Work out the finished part from the listing and answer in its coordinate system (mm). A direction names the side the tool comes from. Coordinates: 2 decimals unless noted, no trailing zeros. Loops run counter-clockwise (first coordinate to the right, second up) from the corner with the lowest first, then second, coordinate; pieces in that order, holes last. Notation, with made-up numbers: (7.25, -34.5) -> (18.25, -34.5) arc R22 ccw to (18.25, -16.5) -> close; hole circle Ø6 at (85.5, 56). An arc over 180 degrees is marked (long way). Use a Markdown table: item, result.
from build123d import *

# Parameters (mm, degrees)
F2_DEPTH = 5
F3_DEPTH = 5
F5_COUNT = 20
F5_ANGLE = 342


with BuildPart() as f2:
    # F1 (on Front) → F2 (new body)
    with BuildSketch(Plane.XZ):
        with BuildLine():
            ThreePointArc((18.791765015, -0.2801004202), (18.7933305583, -0.140054099), (18.7938524157, 0))
            ThreePointArc((18.7938524157, 0), (18.7238802654, 1.6202457939), (18.5144848465, 3.2284267827))
            ThreePointArc((18.5144848465, 3.2284267827), (-18.7354346217, -1.4806681458), (18.791765015, -0.2801004202))
        make_face()
    extrude(amount=F2_DEPTH)

    # F1 (on Front) → F3 (join)
    with BuildSketch(Plane.XZ):
        with BuildLine():
            ThreePointArc((18.5144848465, 3.2284267827), (18.7238802654, 1.6202457939), (18.7938524157, 0))
            ThreePointArc((18.7938524157, 0), (18.7933305583, -0.140054099), (18.791765015, -0.2801004202))
            ThreePointArc((18.791765015, -0.2801004202), (20.4674995965, 0.1731452079), (21.9757526216, 1.0326164403))
            ThreePointArc((21.9757526216, 1.0326164403), (21.9316163904, 1.7332635421), (21.8651473224, 2.4321456718))
            ThreePointArc((21.8651473224, 2.4321456718), (20.2406124153, 3.0440315456), (18.5144848465, 3.2284267827))
        make_face()
    extrude(amount=F3_DEPTH)

    # F5: F2 ×20 about axis
    f5_axis = Axis((0, 6.1465417966, 0), (0, 1, 0))


with BuildPart() as f2_1:
    add(f2.part)
    for i in range(1, F5_COUNT):
        add(f2.part.rotate(f5_axis, i * F5_ANGLE / (F5_COUNT - 1)))


solid = f2_1.part
Q1. Consider line 1 (Z direction, x = -15.5, y = -3.1); line 2 (X direction, y = -2.4, z = -16.5); line 3 (X direction, y = -0.2, z = -1). Determine where each line is inside the solid, lowest interval first. Write a range as [from, to].
Solved:
| item | result |
|---|---|
| line 1 | [-14.67, -10.95], [-10.63, 11.5] |
| line 2 | [-11.85, 9], [12.24, 14.55] |
| line 3 | [-21.93, 18.77] |
Q2. Section A-A on z = 5 is taken. Determine the outline of the cut face in (x, y).
Solved:
| item | result |
|---|---|
| outline | (-21.42, -5) -> (18.12, -5) -> (18.12, 0) -> (-21.42, 0) -> close |
Q3. Given pin 1 Ø12 at (x, z) = (-2, -0.5) entering from +Y; pin 2 Ø3 at (x, y) = (8.5, -1) entering from -Z; pin 3 Ø3 at (x, y) = (5.5, -1) entering from +Z, each flat-ended and moving along its own axis, determine where each tip first touches the part or whether it passes through.
Solved:
| item | result |
|---|---|
| pin 1 | y = 0 |
| pin 2 | z = -20.58 |
| pin 3 | z = 21.55 |
Q4. For faces 1 (the cylindrical face through (-18.277, -2.465, -4.377)), 2 (the cylindrical face through (-14.284, -2.465, 12.214)), 3 (the cylindrical face through (-12.15, -2.465, 16.444)), 4 (the cylindrical face through (-3.37, -2.46, -20.21)), determine the directions among +Z, -Z, +X, -X, +Y, -Y from which every point of the face is accessible in a straight line to the end or side of a thin tool.
Solved:
| item | result |
|---|---|
| face 1 | -X, +Y, -Y |
| face 2 | +Y, -Y |
| face 3 | +Z, +Y, -Y |
| face 4 | -Z, +Y, -Y |
Q5. Determine the mould class of faces 5 (the cylindrical face through (-18.18, -2.46, 9.45)), 6 (the cylindrical face through (14.284, -2.465, -12.214)), 7 (the cylindrical face through (18.757, -2.465, -11.497)), 8 (the cylindrical face through (3.37, -2.46, 20.21)) for opening direction Z: pulls with the +Z half, pulls with the -Z half, needs draft (parallel to the pull), parting line crosses it, or undercut.
Solved:
| item | result |
|---|---|
| face 5 | undercut |
| face 6 | undercut |
| face 7 | pulls with the -Z half |
| face 8 | pulls with the +Z half |
